Model file for the job. Use its own axes, mm. A direction names the side the tool comes from. Coordinates: 2 decimals unless noted, no trailing zeros. Write each loop counter-clockwise with the first axis right and the second up, starting at its lowest first coordinate (ties: lowest second). Pieces come first, ordered by that corner, then holes. Notation, with made-up numbers: M -22,39.25 L 36,39.25 A31 cw 36,69.25 Z; hole C 47,-18.5 d2. An arc over 180 degrees is marked long. Put each result on its own line as item: value. Start each with the question number.
Q1. Cut at B-B (y = 7.5). Write the cut outline in (x, z), then the cut area to 3 significant figures.
Q2. Cut at A-A (y = -1). Write the cut outline in (x, z), then the cut area to 3 significant figures.
Q3. Which spindle directions (+Z, -Z, +X, -X, +Y, -Y) get a long thin tool onto all of the face, cutting with end or side? Do faces 1 (the cylindrical face through (2.847, 3.986, -0.123)), 2 (the cylindrical face through (3.047, 13.605, -0.132)). Say none if no direction does.
Q4. Drill centre lines: line 1 along X through (y, z) = (0, 0); line 2 along Z through (x, y) = (0.05, -1.25); line 3 along Y through (x, z) = (0, 0.5). Where is each one in solid material? Low to high.
Q5. Drop flat-ended pins along their axis: pin 1 (3 mm diameter, centred on x = 1, y = 6, fed in from +Z); pin 2 (1.5 mm diameter, centred on y = 8.5, z = 0.5, fed in from -X); pin 3 (1 mm diameter, centred on x = -1, z = 2, fed in from +Y). Give the stop position or say it passes through.
```python
from build123d import *


with BuildPart() as part:
    # Sketch1 → Revolve1 (revolve)
    with BuildSketch(Plane.XY):
        with BuildLine():
            Line((-2.95, 13.11209092), (-2.75, 13.11209092))
            Line((-2.75, 13.11209092), (-2.75, -4.88790908))
            Line((-2.75, -4.88790908), (-1.55, -4.88790908))
            Line((-1.55, -4.88790908), (-1.55, 2.262295082))
            Line((-1.55, 2.262295082), (0.05, 2.262295082))
            Line((0.05, 2.262295082), (0.05, 16.561580663))
            ThreePointArc((0.05, 16.561580663), (-2.03113883, 16.048582593), (-2.95, 14.11209092))
            Line((-2.95, 14.11209092), (-2.95, 13.11209092))
        make_face()
    revolve(axis=Axis((0.05, 16.561580663, 0), (0, -1, 0)))


solid = part.part
```
Computed values:
1. outline: C 0.05,0 d5.6
1. area: 24.6 mm2
2. outline: C 0.05,0 d5.6; hole C 0.05,0 d3.2
2. area: 16.6 mm2
3. face 1: -Y
3. face 2: +Y, -Y
4. line 1: -2.75 to -1.55, 1.65 to 2.85
4. line 2: -2.8 to -1.6, 1.6 to 2.8
4. line 3: 2.26 to 16.61
5. pin 1: z = 2.8
5. pin 2: x = -2.75
5. pin 3: y = 16.27
